Could you check a few things on this drawing? It's one solid part, dimensions in mm from its lowest x, y, z. A direction names the side the tool comes from. Give positions to 0.01 mm unless a question says otherwise; leave off trailing zeros. Order: outer loops, then holes, each group sorted by start corner. A loop starts at its lowest first (then second) coordinate and runs counter-clockwise, first axis right, second up.
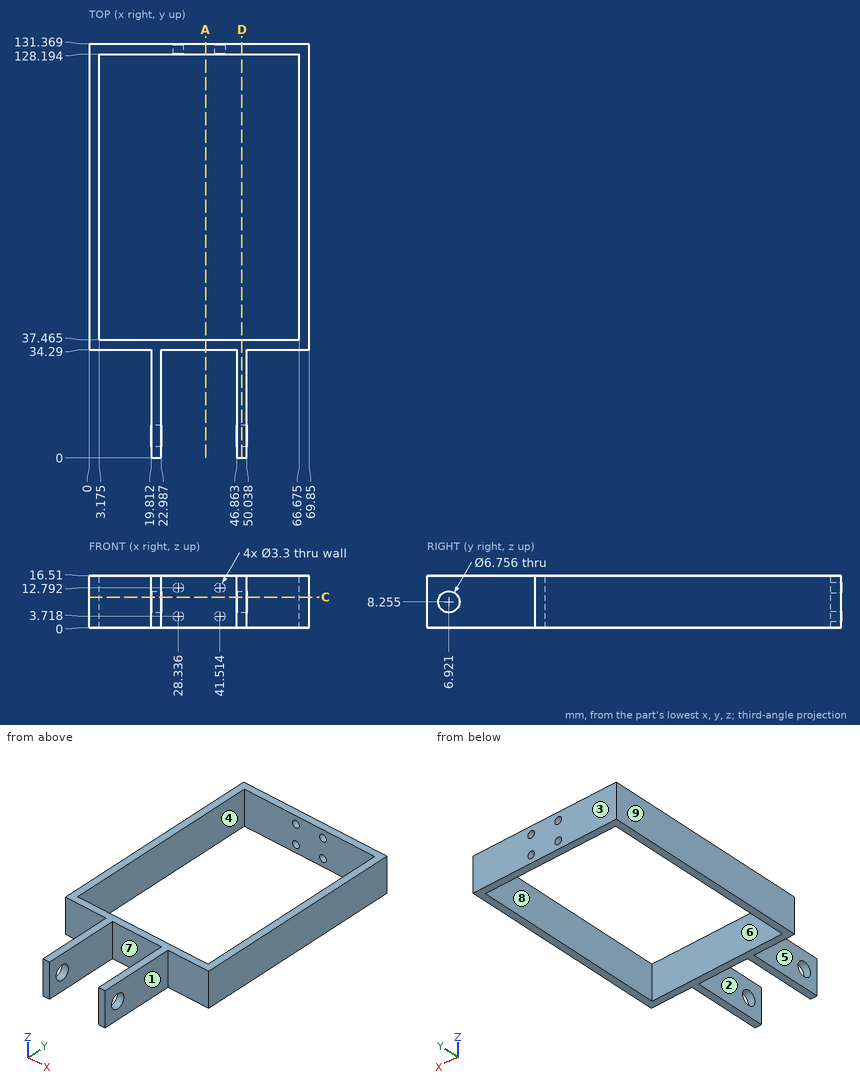
Q1. If we section it at A-A on x = 37: List the corners of the cut face in (y, z) for me (1 decimal).
Filled sheet:
outline: (34.3, 0) - (37.5, 0) - (37.5, 16.5) - (34.3, 16.5) - close; (128.2, 0) - (131.4, 0) - (131.4, 16.5) - (128.2, 16.5) - close
Q2. Thinking about a two-plate mould opening in Y: for the marked faces 6, 7, 8 and 9, which applies, released by +Y, released by -Y, zero draft, split by the parting line, or undercut?
Filled sheet:
face 6: undercut
face 7: released by -Y
face 8: undercut
face 9: zero draft
Q3. I'm going to push flat-ended pins straight in: P1, Ø3, axis at x = 28.34, z = 12.79, coming from the -Y side; P2, Ø4, axis at y = 104.5, z = 2.5, coming from the -X side; P3, Ø1.5, axis at y = 29, z = 11, coming from the +X side; P4, Ø10, axis at x = 9, y = 102, coming from the +Z side. Where does each tip first touch, or does it pass through?
Filled sheet:
P1: stops at y = 34.29
P2: stops at x = 0
P3: stops at x = 50.04
P4: passes through
Q4. If we section it at D-D on x = 48.5: List the corners of the cut face in (y, z) for me (1 decimal).
Filled sheet:
outline: (0, 0) - (37.5, 0) - (37.5, 16.5) - (0, 16.5) - close; (128.2, 0) - (131.4, 0) - (131.4, 16.5) - (128.2, 16.5) - close; hole circle Ø6.8 at (6.9, 8.3)
Q5. If we section it at C-C on z = 9.75: Give the number of separate pieces and of enclosed holes in the cut face, plus the area to 3 significant figures.
Filled sheet:
separate pieces: 3
enclosed holes: 1
area: 1,200 mm2
Q6. For the marked faces 1, 2, 3, 4 and 5, which set-ups out of +Z, -Z, +X, -X, +Y, -Y let a thin tool reach every point of the face, with its end or its side?
Filled sheet:
face 1: +Z, -Z, +X, -Y
face 2: +Z, -Z, -Y
face 3: +Z, -Z, +X, -X, +Y
face 4: +Z, -Z
face 5: +Z, -Z, -X, -Y
Q7. I need wall thicknesses on L1, parallel to X at y = 16.5, z = 2; L2, parallel to Y at x = 33.5, z = 9.75 (1 decimal); L3, parallel to Y at x = 49, z = 2.75 (1 decimal). Which ranges of each line are inside material? Lowest first, please.
Filled sheet:
L1: x = 19.81 to 22.99, 46.86 to 50.04
L2: y = 34.3 to 37.5, 128.2 to 131.4
L3: y = 0 to 37.5, 128.2 to 131.4
